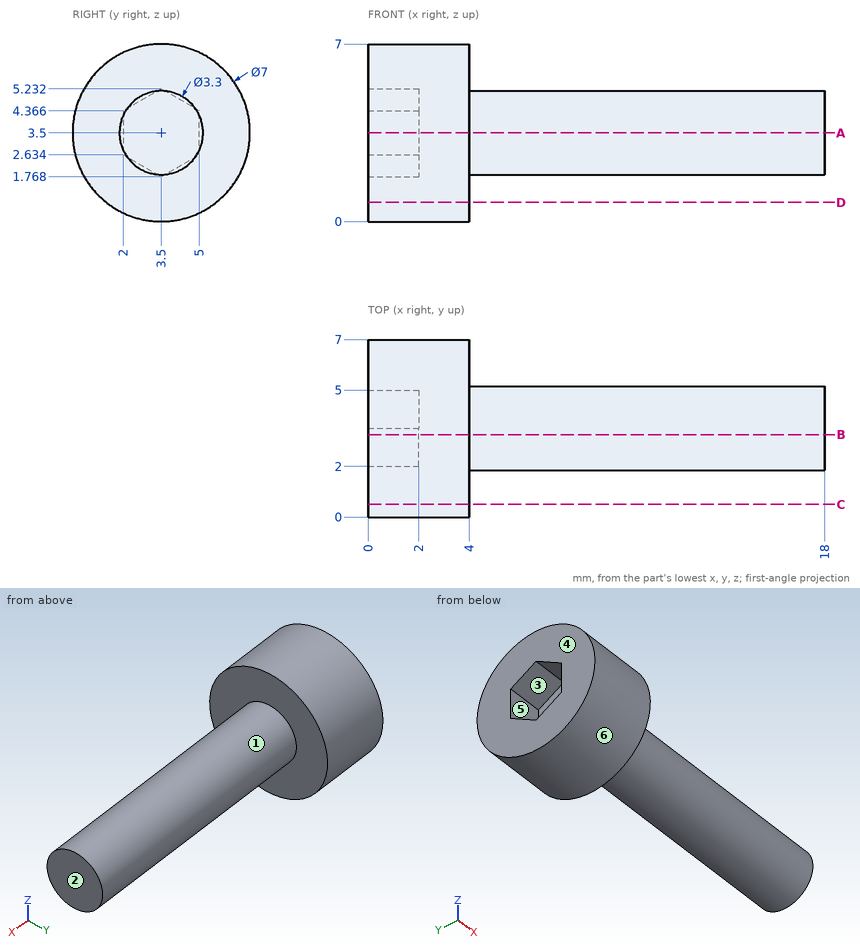
Verification items for this drawing (mm, ordinates from the low corner). A direction names the side the tool comes from. Give positions to 0.01 mm unless a question says otherwise; leave off trailing zeros. Order: outer loops, then holes, each group sorted by start corner. A loop starts at its lowest first (then second) coordinate and runs counter-clockwise, first axis right, second up.
1) Cross-section at A-A (z = 3.5). Record the boundary of the cut face in (x, y).
Results are:
outline: (0, 0) - (4, 0) - (4, 1.85) - (18, 1.85) - (18, 5.15) - (4, 5.15) - (4, 7) - (0, 7) - (0, 5) - (2, 5) - (2, 2) - (0, 2) - close
2) Gauge pin test, flat ends, axial feed: pin 1 (1 mm diameter, centred on y = 4, z = 1.5, fed in from -X); pin 2 (2 mm diameter, centred on x = 14, z = 2, fed in from -Y). Record the tip position at first contact, or that the pin passes through.
Results are:
pin 1: stops at x = 0
pin 2: stops at y = 1.93
3) Cross-section at D-D (z = 0.75). Record the boundary of the cut face in (x, y) (3 decimals), then the cut area to 3 significant figures.
Results are:
outline: (0, 1.335) - (4, 1.335) - (4, 5.665) - (0, 5.665) - close
area: 17.3 mm2
4) Draft check along Y on the marked faces 4, 5 and 6. Enter one of: released by +Y, released by -Y, zero draft, split by the parting line, or undercut.
Results are:
face 4: zero draft
face 5: undercut
face 6: split by the parting line
5) Cross-section at C-C (y = 0.5). Record the boundary of the cut face in (x, z), then the cut area to 3 significant figures.
Results are:
outline: (0, 1.7) - (4, 1.7) - (4, 5.3) - (0, 5.3) - close
area: 14.4 mm2
6) Material ranges on probe 1 along X at (y, z) = (3.5, 1); probe 2 along X at (y, z) = (3.75, 5); probe 3 along Y at (x, z) = (1.25, 2.25) (1 decimal), recorded low to high.
Results are:
probe 1: x = 0 to 4
probe 2: x = 2 to 18
probe 3: y = 0.2 to 2.7, 4.3 to 6.8
7) Cross-section at B-B (y = 3.25). Record the boundary of the cut face in (x, z), then the cut area to 3 significant figures.
Results are:
outline: (0, 0.01) - (4, 0.01) - (4, 1.87) - (18, 1.87) - (18, 5.13) - (4, 5.13) - (4, 6.99) - (0, 6.99) - (0, 5.09) - (2, 5.09) - (2, 1.91) - (0, 1.91) - close
area: 67.2 mm2
8) Tool access check on the marked faces 1, 2 and 3. Record the directions out of +Z, -Z, +X, -X, +Y, -Y that give a thin tool (end or side, any length) a straight path to the whole face; none if there is none.
Results are:
face 1: +X
face 2: +Z, -Z, +X, +Y, -Y
face 3: -X
